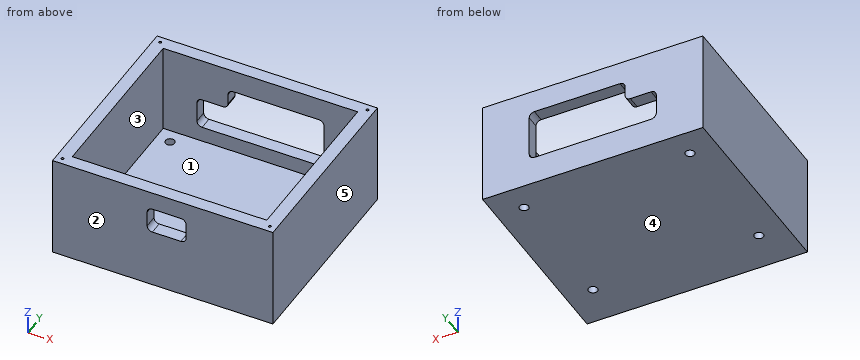
```python
from build123d import *

# Parameters (mm, degrees)
F0_W     = 75
F0_H     = 67
F0_R     = 1.75
F1_DEPTH = 5
F0_W_2   = 85
F0_H_2   = 77
F2_DEPTH = 40
F3_R     = 0.5
F4_DEPTH = 15
F6_DEPTH = 25
F8_DEPTH = 25


with BuildPart() as f1:
    # F0 (on Top) → F1 (new body)
    with BuildSketch(Plane.XY):
        Rectangle(F0_W, F0_H)
        with Locations((-32, -22.8)):
            Circle(F0_R, mode=Mode.SUBTRACT)
        with Locations((32, -22.8)):
            Circle(F0_R, mode=Mode.SUBTRACT)
        with Locations((-32, 28)):
            Circle(F0_R, mode=Mode.SUBTRACT)
        with Locations((32, 28)):
            Circle(F0_R, mode=Mode.SUBTRACT)
    extrude(amount=F1_DEPTH)

    # F0 (on Top) → F2 (join)
    with BuildSketch(Plane.XY):
        Rectangle(F0_W_2, F0_H_2)
        Rectangle(F0_W, F0_H, mode=Mode.SUBTRACT)
    extrude(amount=F2_DEPTH)

    # F3 (on face) → F4 (cut)
    with BuildSketch(Plane.XY.offset(40)):
        with Locations((-40, -36)):
            Circle(F3_R)
        with Locations((-40, 36)):
            Circle(F3_R)
        with Locations((40, -36)):
            Circle(F3_R)
        with Locations((40, 36)):
            Circle(F3_R)
    extrude(amount=-F4_DEPTH, mode=Mode.SUBTRACT)

    # F5 (on face) → F6 (cut)
    with BuildSketch(Plane.XZ.offset(38.5)):
        with BuildLine():
            Line((7, 33), (-4, 33))
            ThreePointArc((-4, 33), (-5.414214, 32.414214), (-6, 31))
            Line((-6, 31), (-6, 25))
            ThreePointArc((-6, 25), (-5.414214, 23.585786), (-4, 23))
            Line((-4, 23), (7, 23))
            ThreePointArc((7, 23), (8.414214, 23.585786), (9, 25))
            Line((9, 25), (9, 31))
            ThreePointArc((9, 31), (8.414214, 32.414214), (7, 33))
        make_face()
    extrude(amount=-F6_DEPTH, mode=Mode.SUBTRACT)

    # F7 (on face) → F8 (cut)
    with BuildSketch(Plane(origin=(0, 38.5, 0), x_dir=(-1, 0, 0), z_dir=(0, 1, 0))):
        with BuildLine():
            Line((10.5, 31), (-22.5, 31))
            ThreePointArc((-22.5, 31), (-23.914214, 30.414214), (-24.5, 29))
            Line((-24.5, 29), (-24.5, 13))
            ThreePointArc((-24.5, 13), (-23.914214, 11.585786), (-22.5, 11))
            Line((-22.5, 11), (22.5, 11))
            ThreePointArc((22.5, 11), (23.914214, 11.585786), (24.5, 13))
            Line((24.5, 13), (24.5, 21))
            ThreePointArc((24.5, 21), (23.914214, 22.414214), (22.5, 23))
            Line((22.5, 23), (14.5, 23))
            ThreePointArc((14.5, 23), (13.085786, 23.585786), (12.5, 25))
            Line((12.5, 25), (12.5, 29))
            ThreePointArc((12.5, 29), (11.914214, 30.414214), (10.5, 31))
        make_face()
    extrude(amount=-F8_DEPTH, mode=Mode.SUBTRACT)


solid = f1.part
```
Read the model definition and answer for the solid it produces. Units are mm, in the model's axes. Face numbers are marked on the shaded views. A direction names the side the tool comes from. Coordinates: 2 decimals unless noted, no trailing zeros. Loops run counter-clockwise (first coordinate to the right, second up) from the corner with the lowest first, then second, coordinate; pieces in that order, holes last.
(1) A tool of negligible diameter and unlimited length cuts with its end or side. For the marked faces 1 and 2, from which of +Z, -Z, +X, -X, +Y, -Y can it reach the whole face along a straight path? Write none if from no direction.
Solution:
face 1: +Z
face 2: +Z, -Z, +X, -X, -Y
(2) The part is cut by section D-D (z = 7). Determine the outline of the cut face in (x, y), and give its area (3 significant figures).
Solution:
outline: (-42.5, -38.5) - (42.5, -38.5) - (42.5, 38.5) - (-42.5, 38.5) - close; hole (-37.5, -33.5) - (37.5, -33.5) - (37.5, 33.5) - (-37.5, 33.5) - close
area: 1,520 mm2
(3) Flat-ended cylindrical pins translate along their axes: pin 1 Ø0.8 at (x, y) = (-40, -36) entering from +Z; pin 2 Ø4.5 at (x, y) = (-32, 28) entering from +Z. Find the tip coordinate at first contact, or state that the pin passes through.
Solution:
pin 1: stops at z = 25
pin 2: stops at z = 5
(4) The mould has two halves that part along X. Classify the marked faces 3, 4 and 5: released by +X, released by -X, zero draft, split by the parting line, or undercut.
Solution:
face 3: undercut
face 4: zero draft
face 5: released by +X
(5) Consider line 1 along Y through (x, z) = (-32, 3.95); line 2 along Y through (x, z) = (40, 33); line 3 along Z through (x, y) = (19, 35). Determine where each line is inside the solid, lowest interval first.
Solution:
line 1: y = -38.5 to -24.55, -21.05 to 26.25, 29.75 to 38.5
line 2: y = -38.5 to -36.5, -35.5 to 35.5, 36.5 to 38.5
line 3: z = 0 to 11, 31 to 40
(6) The part is cut by section C-C (z = 30). Determine the outline of the cut face in (x, y).
Solution:
outline: (-42.5, -38.5) - (-6, -38.5) - (-6, -33.5) - (-37.5, -33.5) - (-37.5, 33.5) - (-12.23, 33.5) - (-12.23, 38.5) - (-42.5, 38.5) - close; (9, -38.5) - (42.5, -38.5) - (42.5, 38.5) - (24.23, 38.5) - (24.23, 33.5) - (37.5, 33.5) - (37.5, -33.5) - (9, -33.5) - close; hole circle Ø1 at (-40, -36); hole circle Ø1 at (-40, 36); hole circle Ø1 at (40, -36); hole circle Ø1 at (40, 36)
(7) The part is cut by section B-B (y = -22.8). Determine the outline of the cut face in (x, z).
Solution:
outline: (-42.5, 0) - (-33.75, 0) - (-33.75, 5) - (-37.5, 5) - (-37.5, 40) - (-42.5, 40) - close; (-30.25, 0) - (30.25, 0) - (30.25, 5) - (-30.25, 5) - close; (33.75, 0) - (42.5, 0) - (42.5, 40) - (37.5, 40) - (37.5, 5) - (33.75, 5) - close
(8) The part is cut by section A-A (x = 32). Determine the outline of the cut face in (y, z).
Solution:
outline: (-38.5, 0) - (-24.55, 0) - (-24.55, 5) - (-33.5, 5) - (-33.5, 40) - (-38.5, 40) - close; (-21.05, 0) - (26.25, 0) - (26.25, 5) - (-21.05, 5) - close; (29.75, 0) - (38.5, 0) - (38.5, 40) - (33.5, 40) - (33.5, 5) - (29.75, 5) - close
